Geometry check sheet. Reference: the model listing, model coordinates, mm. Face numbers are marked on the shaded views. A direction names the side the tool comes from. Coordinates: 2 decimals unless noted, no trailing zeros. Write each loop counter-clockwise with the first axis right and the second up, starting at its lowest first coordinate (ties: lowest second). Pieces come first, ordered by that corner, then holes. Notation, with made-up numbers: (37, 72) -> (49, 72) arc R15 cw to (49, 92) -> close; hole circle Ø3 at (12.25, 27.5). An arc over 180 degrees is marked (long way). Answer in a Markdown table with one row per item. Add a question column.
Q1. Section check A-A, the plane y = -19.25. Record the boundary of the cut face in (x, z), and give its area (3 significant figures).
Q2. Release check for a two-part mould opening along Z. For the marked faces 4, 5, 6 and 7 record: pulls with the +Z half, pulls with the -Z half, needs draft (parallel to the pull), parting line crosses it, or undercut.
Q3. Section check C-C, the plane z = 13.5. Record the boundary of the cut face in (x, y), and give its area (3 significant figures).
Q4. Thickness scan on line 1 (Z direction, x = -18, y = -9.5); line 2 (Y direction, x = -1, z = 23.5); line 3 (Z direction, x = -50, y = -23.5). Record the ranges inside material, lowest first.
Q5. Tool access check on the marked faces 1, 2 and 3. Record the directions out of +Z, -Z, +X, -X, +Y, -Y that give a thin tool (end or side, any length) a straight path to the whole face; none if there is none.
Q6. Gauge pin test, flat ends, axial feed: P1, Ø11.5, axis at x = 17.5, y = -21, coming from the +Z side; P2, Ø7.5, axis at y = -11.5, z = 7, coming from the +X side; P3, Ø5, axis at y = -23, z = 45, coming from the +X side; P4, Ø4, axis at x = 33.5, z = 6, coming from the -Y side. Record the tip position at first contact, or that the pin passes through.
Q7. Section check B-B, the plane x = -5. Record the boundary of the cut face in (y, z), and give its area (3 significant figures).
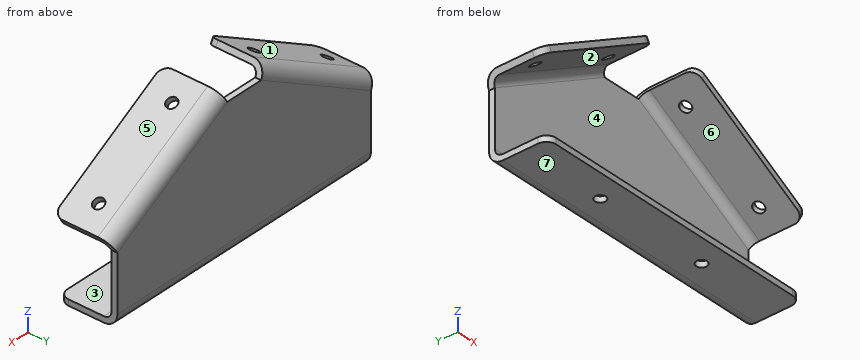
```python
from build123d import *

# Parameters (mm, degrees)
ODGI_CIE_BAZOWE1_DEPTH        = 75
WYTNIJ_WYCI_GNI_CIE1_DEPTH    = 10
ODGI_CIE_KRAW_DZI1_DEPTH      = 75.055534995
ODGI_CIE_KRAW_DZI1_BEND_DEPTH = 75.055534995
OTW_R_POD_RUB_M52_D           = 5.5
OTW_R_POD_RUB_M52_DEPTH       = 10
OTW_R_POD_RUB_M52_TIP         = 1.652366702
OTW_R_POD_RUB_M51_AT_2_COUNT  = 2
OTW_R_POD_RUB_M51_AT_2_PITCH  = 50
ZAOKR_GLENIE1_R               = 5


# Sheet-metal steps are written as plain solids
with BuildPart() as part:
    # Szkic1 → Odgięcie bazowe1 (new, symmetric)
    with BuildSketch(Plane(origin=(0, 0, 0), x_dir=(0, 0, -1), z_dir=(1, 0, 0))):
        with BuildLine():
            Line((0, -27), (0, -4))
            ThreePointArc((0, -4), (-1.171572875, -1.171572875), (-4, 0))
            Line((-4, 0), (-70, 0))
            Line((-70, 0), (-70, 3))
            Line((-70, 3), (-4, 3))
            ThreePointArc((-4, 3), (0.949747468, 0.949747468), (3, -4))
            Line((3, -4), (3, -27))
            Line((3, -27), (0, -27))
        make_face()
    extrude(amount=ODGI_CIE_BAZOWE1_DEPTH, both=True)

    # Szkic6 → Wytnij-wyciągnięcie1 (cut)
    with BuildSketch(Plane(origin=(0, 3, 0), x_dir=(1, 0, 0), z_dir=(0, 1, 0))):
        Polygon((-75, -32.472232503), (-10, -70), (-75, -70), align=None)
        Polygon((75, -70), (75, -32.472232503), (10, -70), align=None)
    extrude(amount=-WYTNIJ_WYCI_GNI_CIE1_DEPTH, mode=Mode.SUBTRACT)

    # Odgięcie krawędzi1 section (across the edge) → Odgięcie krawędzi1 (add)
    with BuildSketch(Plane(origin=(-12, 0, 73.464101615), x_dir=(0.4999999999999948, -3.3854238149706416e-15, -0.8660254037844417), z_dir=(-0.8660254037844417, 0, -0.4999999999999948))):
        with BuildLine():
            Line((-3, 4), (-3, 27))
            Line((-3, 27), (0, 27))
            Line((0, 27), (0, 4))
            ThreePointArc((0, 4), (1.171572875, 1.171572875), (4, 0))
            Line((4, 0), (4, -3))
            ThreePointArc((4, -3), (-0.949747468, -0.949747468), (-3, 4))
        make_face()
    extrude(amount=ODGI_CIE_KRAW_DZI1_DEPTH)

    # Odgięcie krawędzi1 section 2 (across the edge) → Odgięcie krawędzi1 bend (add)
    with BuildSketch(Plane(origin=(77, 0, 35.936334118), x_dir=(-0.49999999999999467, -3.3854238149706423e-15, -0.8660254037844417), z_dir=(-0.8660254037844417, 0, 0.49999999999999467))):
        with BuildLine():
            Line((-3, 4), (-3, 27))
            Line((-3, 27), (0, 27))
            Line((0, 27), (0, 4))
            ThreePointArc((0, 4), (1.171572875, 1.171572875), (4, 0))
            Line((4, 0), (4, -3))
            ThreePointArc((4, -3), (-0.949747468, -0.949747468), (-3, 4))
        make_face()
    extrude(amount=ODGI_CIE_KRAW_DZI1_BEND_DEPTH)

    # Otwór pod śrubę M52
    with Locations(Plane(origin=(0, 0, -3), x_dir=(-1, 0, 0), z_dir=(0, 0, -1))):
        with Locations((-30, -15), (30, -15)):
            Hole(OTW_R_POD_RUB_M52_D / 2, depth=OTW_R_POD_RUB_M52_DEPTH)
            with Locations((0, 0, -(OTW_R_POD_RUB_M52_DEPTH + OTW_R_POD_RUB_M52_TIP / 2))):  # 118° drill point
                Cone(0, OTW_R_POD_RUB_M52_D / 2, OTW_R_POD_RUB_M52_TIP, mode=Mode.SUBTRACT)

    # Szkic16 → Otwór pod śrubę M51 (revolve, cut)
    with BuildSketch(Plane(origin=(-67.650635095, -13, 44.798294078), x_dir=(0.8660254037844417, 0, 0.4999999999999949), z_dir=(0, 1, 0))):
        Polygon((0, 0), (0, 11.652366702), (2.75, 10), (2.75, 0), align=None)
    otw_r_pod_rub_m51 = revolve(axis=Axis((-70.825635095, -13, 50.297555392), (0.4999999999999949, -3.3879771740092313e-15, -0.8660254037844417)), mode=Mode.SUBTRACT)

    # Otwór pod śrubę M51 at 2: Otwór pod śrubę M51 ×2
    with Locations(*[Vector(0.8660254037844417, 1.9224128461953825e-15, 0.49999999999999495) * (i * OTW_R_POD_RUB_M51_AT_2_PITCH) for i in range(1, OTW_R_POD_RUB_M51_AT_2_COUNT)]):
        add(otw_r_pod_rub_m51, mode=Mode.SUBTRACT)

    # Lustro1: Otwór pod śrubę M51 across plane
    add(otw_r_pod_rub_m51.mirror(Plane(origin=(0, 0, 0), x_dir=(0, 0, 1), z_dir=(1, 0, 0))), mode=Mode.SUBTRACT)

    # Lustro1 copy 1 sketch → Lustro1 copy 1 (revolve, cut)
    with BuildSketch(Plane(origin=(24.349364905, -13, 69.798294078), x_dir=(-0.8660254037844417, 0, 0.4999999999999949), z_dir=(0, 1, 0))):
        Polygon((0, 0), (0, -11.652366702), (2.75, -10), (2.75, 0), align=None)
    revolve(axis=Axis((27.524364905, -13, 75.297555392), (0.4999999999999949, 3.3879771740092313e-15, 0.8660254037844417)), mode=Mode.SUBTRACT)

    # Zaokrąglenie1
    zaokr_glenie1_edges = [part.edges().sort_by_distance(p)[0] for p in [
        (75, -27, -1.5),
        (-12.75, -27, 74.763139721),
        (-77.75, -27, 37.235372223),
        (-75, -27, -1.5),
        (77.75, -27, 37.235372223),
        (12.75, -27, 74.763139721),
    ]]
    fillet(zaokr_glenie1_edges, radius=ZAOKR_GLENIE1_R)


solid = part.part
```
Calculated:
| question | item | result |
|---|---|---|
| 1 | outline | (-78.5, 38.53) -> (-77, 35.94) -> (-12, 73.46) -> (-13.5, 76.06) -> close; (-75, -3) -> (75, -3) -> (75, 0) -> (-75, 0) -> close; (12, 73.46) -> (77, 35.94) -> (78.5, 38.53) -> (13.5, 76.06) -> close |
| 1 | area | 900 mm² |
| 2 | face 4 | undercut |
| 2 | face 5 | pulls with the +Z half |
| 2 | face 6 | undercut |
| 2 | face 7 | pulls with the -Z half |
| 3 | outline | (-75, 0) -> (75, 0) -> (75, 3) -> (-75, 3) -> close |
| 3 | area | 450 mm² |
| 4 | line 1 | z = -3 to 0, 70 to 73.46 |
| 4 | line 2 | y = 0 to 3 |
| 4 | line 3 | z = -3 to 0, 51.52 to 54.99 |
| 5 | face 1 | +Z, -X, +Y, -Y |
| 5 | face 2 | -Y |
| 5 | face 3 | +X, -X, -Y |
| 6 | P1 | stops at z = 76.06 |
| 6 | P2 | passes through |
| 6 | P3 | stops at x = 71.63 |
| 6 | P4 | stops at y = 0 |
| 7 | outline | (-27, -3) -> (-4, -3) arc R7 ccw to (3, 4) -> (3, 70) -> (0, 70) -> (0, 4) arc R4 cw to (-4, 0) -> (-27, 0) -> close |
| 7 | area | 293 mm² |
